from build123d import *

# Parameters (mm, degrees)
SKETCH1_W            = 64
SKETCH1_H            = 48
BOSS_EXTRUDE1_DEPTH  = 4
CUT_EXTRUDE1_DEPTH   = 2.4
CUT_EXTRUDE2_DEPTH   = 2.4
BOSS_EXTRUDE3_DEPTH  = 50
BOSS_EXTRUDE4_DEPTH  = 50
SKETCH10_W           = 2.02372337
SKETCH10_H           = 15.25
SKETCH10_W_2         = 25.5
SKETCH10_H_2         = 25.5
CUT_EXTRUDE4_DEPTH   = 9.5
SKETCH13_W           = 36.946258726
SKETCH13_H           = 1
CUT_EXTRUDE6_DEPTH   = 32
SKETCH15_R           = 3.25
BOSS_EXTRUDE5_DEPTH  = 4
CUT_EXTRUDE7_DEPTH   = 7
SKETCH18_W           = 5.8
SKETCH18_H           = 2.6
CUT_EXTRUDE8_DEPTH   = 5
SKETCH19_R           = 1.75
BOSS_EXTRUDE8_DEPTH  = 4.4
FILLET1_R            = 1.5
SKETCH20_R           = 2
BOSS_EXTRUDE9_DEPTH  = 4
FILLET2_R            = 3
SKETCH22_R           = 1.75
CUT_EXTRUDE9_DEPTH   = 2
SKETCH23_R           = 2.5
CUT_EXTRUDE10_DEPTH  = 3
SKETCH24_W           = 2
SKETCH24_H           = 10
BOSS_EXTRUDE10_DEPTH = 4
SKETCH25_W           = 2
SKETCH25_H           = 10
BOSS_EXTRUDE11_DEPTH = 13
SKETCH26_W           = 2
SKETCH26_H           = 10
BOSS_EXTRUDE12_DEPTH = 4
FILLET4_R            = 1


with BuildPart() as part:
    # Sketch1 → Boss-Extrude1 (new body)
    with BuildSketch(Plane(origin=(0, 0, 0), x_dir=(1, 0, 0), z_dir=(0, 1, 0))):
        Rectangle(SKETCH1_W, SKETCH1_H)
    extrude(amount=BOSS_EXTRUDE1_DEPTH)

    # Sketch2 → Cut-Extrude1 (cut)
    with BuildSketch(Plane.XZ):
        Polygon((-20.651368439, -16), (-22.325684219, -13.1), (-25.674315781, -13.1), (-27.348631561, -16), (-25.674315781, -18.9), (-22.325684219, -18.9), align=None)
    extrude(amount=-CUT_EXTRUDE1_DEPTH, mode=Mode.SUBTRACT)

    # Sketch4 → Cut-Extrude2 (cut)
    with BuildSketch(Plane.XZ):
        Polygon((9.348631561, 10), (7.674315781, 12.9), (4.325684219, 12.9), (2.651368439, 10), (4.325684219, 7.1), (7.674315781, 7.1), align=None)
    extrude(amount=-CUT_EXTRUDE2_DEPTH, mode=Mode.SUBTRACT)

    # Sketch6 → Boss-Extrude3 (add)
    with BuildSketch(Plane(origin=(0, 4, 0), x_dir=(1, 0, 0), z_dir=(0, 1, 0))):
        Polygon((-29, -21), (-29, 21), (-29, 24), (-32, 24), (-32, -24), (32, -24), (32, 24), (29, 24), (29, 21), (29, -21), align=None)
    extrude(amount=BOSS_EXTRUDE3_DEPTH)

    # Sketch9 → Boss-Extrude4 (add)
    with BuildSketch(Plane(origin=(0, 4, 0), x_dir=(1, 0, 0), z_dir=(0, 1, 0))):
        Polygon((29, -13), (1, -13), (-7, -21), (29, -21), align=None)
    extrude(amount=BOSS_EXTRUDE4_DEPTH)

    # Sketch10 → Cut-Extrude4 (cut)
    with BuildSketch(Plane(origin=(0, 0, 13), x_dir=(-1, 0, 0), z_dir=(0, 0, -1))):
        with Locations((-14, 46.375)):
            Rectangle(SKETCH10_W, SKETCH10_H)
        with Locations((-14, 26)):
            Rectangle(SKETCH10_W_2, SKETCH10_H_2)
    extrude(amount=-CUT_EXTRUDE4_DEPTH, mode=Mode.SUBTRACT)

    # Sketch13 → Cut-Extrude6 (cut)
    with BuildSketch(Plane(origin=(0, 54, 0), x_dir=(1, 0, 0), z_dir=(0, 1, 0))):
        with Locations((10.526870637, -13.5)):
            Rectangle(SKETCH13_W, SKETCH13_H)
    extrude(amount=-CUT_EXTRUDE6_DEPTH, mode=Mode.SUBTRACT)

    # Sketch15 → Boss-Extrude5 (add)
    with BuildSketch(Plane(origin=(0, 54, 0), x_dir=(1, 0, 0), z_dir=(0, 1, 0))):
        Polygon((-29, -1), (-9, -21), (-29, -21), align=None)
        with Locations((-23, -15)):
            Circle(SKETCH15_R, mode=Mode.SUBTRACT)
    extrude(amount=-BOSS_EXTRUDE5_DEPTH)

    # Sketch17 → Cut-Extrude7 (cut)
    with BuildSketch(Plane(origin=(0, 54, 0), x_dir=(1, 0, 0), z_dir=(0, 1, 0))):
        Polygon((24, -15.651368439), (21.1, -17.325684219), (21.1, -20.674315781), (24, -22.348631561), (26.9, -20.674315781), (26.9, -17.325684219), align=None)
    extrude(amount=-CUT_EXTRUDE7_DEPTH, mode=Mode.SUBTRACT)

    # Sketch18 → Cut-Extrude8 (cut)
    with BuildSketch(Plane(origin=(0, 0, 14), x_dir=(-1, 0, 0), z_dir=(0, 0, -1))):
        with Locations((-24, 48.3)):
            Rectangle(SKETCH18_W, SKETCH18_H)
    extrude(amount=-CUT_EXTRUDE8_DEPTH, mode=Mode.SUBTRACT)

    # Sketch19 → Boss-Extrude8 (add)
    with BuildSketch(Plane(origin=(0, 54, 0), x_dir=(1, 0, 0), z_dir=(0, 1, 0))):
        Polygon((24, -15.651368439), (26.9, -17.325684219), (26.9, -20.674315781), (24, -22.348631561), (21.1, -20.674315781), (21.1, -17.325684219), align=None)
        with Locations((24, -19)):
            Circle(SKETCH19_R, mode=Mode.SUBTRACT)
    extrude(amount=-BOSS_EXTRUDE8_DEPTH)

    # Fillet1
    fillet1_edges = [part.edges().sort_by_distance(p)[0] for p in [
        (-29, 50, 11),
        (-19, 50, 21),
    ]]
    fillet(fillet1_edges, radius=FILLET1_R)

    # Sketch20 → Boss-Extrude9 (add)
    with BuildSketch(Plane.XZ):
        with BuildLine():
            Line((43.102082828, 12.467708073), (32.000000003, 23.999999995))
            Line((32.000000003, 23.999999995), (32, -6.000000006))
            Line((32, -6.000000006), (43.102082819, 5.532291906))
            ThreePointArc((43.102082819, 5.532291906), (44.500000003, 8.999999988), (43.102082828, 12.467708073))
        make_face()
        with Locations((39.500000002, 8.999999994)):
            Circle(SKETCH20_R, mode=Mode.SUBTRACT)
        with BuildLine():
            Line((-32, -24), (-32, 2.000000002))
            Line((-32, 2.000000002), (-42.978939192, -7.408763151))
            ThreePointArc((-42.978939192, -7.408763151), (-44.499999999, -10.999999999), (-42.978939192, -14.591236846))
            Line((-42.978939192, -14.591236846), (-32, -24))
        make_face()
        with Locations((-39.499999999, -10.999999999)):
            Circle(SKETCH20_R, mode=Mode.SUBTRACT)
    extrude(amount=-BOSS_EXTRUDE9_DEPTH)

    # Fillet2
    fillet2_edges = [part.edges().sort_by_distance(p)[0] for p in [
        (-32, 4, -10.999999999),
        (32.000000002, 4, 8.999999995),
    ]]
    fillet(fillet2_edges, radius=FILLET2_R)

    # Sketch22 → Cut-Extrude9 (cut)
    with BuildSketch(Plane.XZ.offset(-2.4)):
        with Locations((-24, -16)):
            Circle(SKETCH22_R)
        with Locations((6, 10)):
            Circle(SKETCH22_R)
    extrude(amount=-CUT_EXTRUDE9_DEPTH, mode=Mode.SUBTRACT)

    # Sketch23 → Cut-Extrude10 (cut)
    with BuildSketch(Plane(origin=(0, 0, 22.5), x_dir=(-1, 0, 0), z_dir=(0, 0, -1))):
        with Locations((-22.485281374, 34.485281374)):
            Circle(SKETCH23_R)
        with Locations((-5.514718626, 34.485281374)):
            Circle(SKETCH23_R)
        with Locations((-5.514718626, 17.514718626)):
            Circle(SKETCH23_R)
        with Locations((-22.485281374, 17.514718626)):
            Circle(SKETCH23_R)
        with Locations((-22.485281374, 26)):
            Circle(SKETCH23_R)
        with Locations((-5.514718626, 26)):
            Circle(SKETCH23_R)
        with BuildLine():
            Line((-11, 30), (-11, 22))
            ThreePointArc((-11, 22), (-14, 19), (-17, 22))
            Line((-17, 22), (-17, 30))
            ThreePointArc((-17, 30), (-14, 33), (-11, 30))
        make_face()
    extrude(amount=-CUT_EXTRUDE10_DEPTH, mode=Mode.SUBTRACT)

    # Sketch24 → Boss-Extrude10 (add)
    with BuildSketch(Plane.ZY.offset(-29)):
        with Locations((9, 27)):
            Rectangle(SKETCH24_W, SKETCH24_H)
    extrude(amount=BOSS_EXTRUDE10_DEPTH)

    # Sketch25 → Boss-Extrude11 (add)
    with BuildSketch(Plane(origin=(0, 0, 21), x_dir=(-1, 0, 0), z_dir=(0, 0, -1))):
        with Locations((2, 27)):
            Rectangle(SKETCH25_W, SKETCH25_H)
    extrude(amount=BOSS_EXTRUDE11_DEPTH)

    # Sketch26 → Boss-Extrude12 (add)
    with BuildSketch(Plane(origin=(-1, 0, 0), x_dir=(0, 0, -1), z_dir=(1, 0, 0))):
        with Locations((-9, 27)):
            Rectangle(SKETCH26_W, SKETCH26_H)
    extrude(amount=BOSS_EXTRUDE12_DEPTH)

    # Fillet4
    fillet4_edges = [part.edges().sort_by_distance(p)[0] for p in [
        (27, 32, 8),
        (27, 22, 8),
        (25, 32, 9),
        (25, 27, 8),
        (25, 22, 9),
        (-3, 22, 12.5),
        (-3, 32, 12.5),
        (-3, 27, 8),
        (0, 32, 8),
        (0, 22, 8),
        (3, 27, 8),
        (3, 32, 9),
        (3, 22, 9),
    ]]
    fillet(fillet4_edges, radius=FILLET4_R)


solid = part.part
CAD build for the part. Positions are in the model's coordinates, mm. A direction names the side the tool comes from. Round coordinates to 2 decimals unless told otherwise and drop trailing zeros. Loops run counter-clockwise (first coordinate to the right, second up) from the corner with the lowest first, then second, coordinate; pieces in that order, holes last.
(1) Cut at D-D (y = 40.5). Give the cut face in (x, z), plus the area to 3 significant figures.
(2) Cut at C-C (x = -24). Give the cut face in (y, z), plus the area to 3 significant figures.
(3) Cut at B-B (y = 10). Give the cut face in (x, z), plus the area to 3 significant figures.
(4) Cut at A-A (x = 14). Give the cut face in (y, z), plus the area to 3 significant figures.
(5) Drop flat-ended pins along their axis: pin 1 (1.2 mm diameter, centred on y = 26.5, z = 23, fed in from -X); pin 2 (3 mm diameter, centred on x = -12.5, y = 20, fed in from -Z); pin 3 (1.5 mm diameter, centred on x = 27.5, y = 26, fed in from -Z). Give the stop position or say it passes through.
(6) Wall check: line 1 along X through (y, z) = (13, 14); line 2 along Y through (x, z) = (16, 21); line 3 along X through (y, z) = (20, 10). Give the ranges that are in metal, low to high.
(7) Two-plate mould, pull along X, no slides. Class faces 1 (the flat face through (0, 27, 24)), 2 (the flat face through (-32, 27, 0)), 3 (the flat face through (0, 4, -2)): +X half, -X half, draft (parallel to the pull), parting line (faces both ways), or undercut.
(8) Which spindle directions (+Z, -Z, +X, -X, +Y, -Y) get a long thin tool onto all of the face, cutting with end or side? Do faces 4 (the flat face through (3.477, 1.183, 8.57)), 5 (the flat face through (26.75, 26, 18)), 6 (the cylindrical face through (22.71, 51.83, 17.82)), 7 (the flat face through (22.53, 48.32, 21.5)). Say none if no direction does.
Findings below:
1. outline: (-32, -24) - (-29, -24) - (-29, 21) - (-7, 21) - (0, 14) - (12.99, 14) - (12.99, 22.5) - (15.01, 22.5) - (15.01, 14) - (29, 14) - (29, -24) - (32, -24) - (32, 24) - (-32, 24) - close
1. area: 672 mm2
2. outline: (0, -24) - (4, -24) - (4, -17.75) - (2.4, -17.75) - (2.4, -18.9) - (0, -18.9) - close; (0, -13.1) - (2.4, -13.1) - (2.4, -14.25) - (4, -14.25) - (4, 21) - (48.5, 21) arc R1.5 cw to (50, 19.5) - (50, 18.09) - (54, 18.09) - (54, 24) - (0, 24) - close; (50, 6) - (54, 6) - (54, 11.91) - (50, 11.91) - close
2. area: 358 mm2
3. outline: (-32, -24) - (-29, -24) - (-29, 21) - (-7, 21) - (1, 13) - (29, 13) - (29, -24) - (32, -24) - (32, 24) - (-32, 24) - close
3. area: 718 mm2
4. outline: (0, -24) - (4, -24) - (4, 13) - (13.25, 13) - (13.25, 22.5) - (19, 22.5) - (19, 24) - (0, 24) - close; (33, 22.5) - (54, 22.5) - (54, 24) - (33, 24) - close
4. area: 334 mm2
5. pin 1: stops at x = -32
5. pin 2: stops at z = 21
5. pin 3: stops at z = 8
6. line 1: x = -32 to -29, 0 to 32
6. line 2: y = 0 to 13.25, 38.75 to 54
6. line 3: x = -32 to -29, 29 to 32
7. face 1: draft
7. face 2: -X half
7. face 3: undercut
8. face 4: -Y
8. face 5: none
8. face 6: +Y
8. face 7: -Z
